Source: CAD feature listing. Evaluate the final solid. Frame: model axes, mm. Face numbers are marked on the shaded views. A direction names the side the tool comes from. Coordinates: 2 decimals unless noted, no trailing zeros. Loops run counter-clockwise (first coordinate to the right, second up) from the corner with the lowest first, then second, coordinate; pieces in that order, holes last. Notation, with made-up numbers: (40, 9) -> (54, 9) arc R17 ccw to (54, 28) -> close; hole circle Ø5 at (77, 71). An arc over 180 degrees is marked (long way). Answer as a JSON object with one key per item and string values. Group by question number.
from build123d import *

# Parameters (mm, degrees)
SKETCH_1_W          = 70.6
SKETCH_1_H          = 84.6
EXTRUDE_1_DEPTH     = 23
SKETCH_2_W          = 18
SKETCH_2_H          = 4.7
EXTRUDE_2_DEPTH     = 2
SKETCH_3_W          = 70.6
SKETCH_3_H          = 3.2
EXTRUDE_5_DEPTH     = 10
CUT_EXTRUDE_START   = -2
SKETCH_4_R          = 11
CUT_EXTRUDE_1_DEPTH = 115.979827321
EXTRUDE_START       = -2
EXTRUDE_1_2_DEPTH   = 2
DELETE_START        = 91
DELETE_FACE_1_DEPTH = 2
CUT_EXTRUDE_2_DEPTH = 43
EXTRUDE_START_2     = 24
EXTRUDE_6_DEPTH     = 2
FILLET_1_R          = 5


# Read off the part's stored shape, not the designer's step: 删除面1
with BuildPart() as part:
    # 草图1 → Extrude 1 (new body)
    with BuildSketch(Plane.XY):
        with Locations((-38.5, 47.5)):
            Rectangle(SKETCH_1_W, SKETCH_1_H)
    extrude(amount=-EXTRUDE_1_DEPTH)

    # 草图2 → 凸台-拉伸2 (add)
    with BuildSketch(Plane(origin=(0, 0, -23), x_dir=(-1, 0, 0), z_dir=(0, 0, -1))):
        with Locations((12.2, 2.85)):
            Rectangle(SKETCH_2_W, SKETCH_2_H)
        with Locations((64.8, 2.85)):
            Rectangle(SKETCH_2_W, SKETCH_2_H)
    extrude(amount=-EXTRUDE_2_DEPTH)

    # 草图3 → 凸台-拉伸5 (add)
    with BuildSketch(Plane(origin=(0, 0, -23), x_dir=(-1, 0, 0), z_dir=(0, 0, -1))):
        with Locations((38.5, 91.4)):
            Rectangle(SKETCH_3_W, SKETCH_3_H)
    extrude(amount=-EXTRUDE_5_DEPTH)

    # 草图4 → 切除-拉伸1 (cut, through all)
    with BuildSketch(Plane.XZ.offset(-5.2).offset(CUT_EXTRUDE_START)):
        with Locations((-60.8, -25)):
            Circle(SKETCH_4_R)
    extrude(amount=-CUT_EXTRUDE_1_DEPTH, mode=Mode.SUBTRACT)

    # 草图5 → Extrude 1 2 (add)
    with BuildSketch(Plane(origin=(0, 93, 0), x_dir=(1, 0, 0), z_dir=(0, 1, 0)).offset(EXTRUDE_START)):
        with BuildLine():
            ThreePointArc((-71.616653826, 23), (-60.8, 14), (-49.983346174, 23))
            Line((-49.983346174, 23), (-51.950010506, 23.363636364))
            ThreePointArc((-51.950010506, 23.363636364), (-60.8, 16), (-69.649989494, 23.363636364))
            Line((-69.649989494, 23.363636364), (-71.616653826, 23))
        make_face()
    extrude(amount=EXTRUDE_1_2_DEPTH)

    # Delete Face 1 outline → Delete Face 1 (cut)
    with BuildSketch(Plane(origin=(0, 0, 0), x_dir=(1, 0, 0), z_dir=(0, 1, 0)).offset(DELETE_START)):
        with BuildLine():
            ThreePointArc((-51.950010506, 23.363636364), (-51.985647631, 23.181431245), (-52.025035613, 23))
            Line((-52.025035613, 23), (-49.983346174, 23))
            Line((-49.983346174, 23), (-51.950010506, 23.363636364))
        make_face()
        with BuildLine():
            Line((-69.649989494, 23.363636364), (-71.616653826, 23))
            Line((-71.616653826, 23), (-69.574964387, 23))
            ThreePointArc((-69.574964387, 23), (-69.614352369, 23.181431245), (-69.649989494, 23.363636364))
        make_face()
    extrude(amount=DELETE_FACE_1_DEPTH, mode=Mode.SUBTRACT)

    # 草图6 → 切除-拉伸2 (cut)
    with BuildSketch(Plane(origin=(-3.2, 0, 0), x_dir=(0, 0, -1), z_dir=(1, 0, 0)).offset(CUT_EXTRUDE_START)):
        Polygon((23, 93), (15, 93), (15, 87.8), (2, 87.8), (2, 7.2), (23, 7.2), align=None)
    extrude(amount=-CUT_EXTRUDE_2_DEPTH, mode=Mode.SUBTRACT)

    # 草图7 → 凸台-拉伸6 (add)
    with BuildSketch(Plane.ZY.offset(5.2).offset(EXTRUDE_START_2)):
        Polygon((-23, 93), (-23, 7.2), (-2, 7.2), (-2, 87.8), (-15, 87.8), (-15, 93), align=None)
    extrude(amount=EXTRUDE_6_DEPTH)

    # 圆角1
    fillet_1_edges = [part.edges().sort_by_distance(p)[0] for p in [
        (-71.687482193, 93, -23),
        (-50.112517807, 93, -23),
        (-30.2, 93, -23),
        (-4.2, 93, -23),
    ]]
    fillet(fillet_1_edges, radius=FILLET_1_R)


solid = part.part
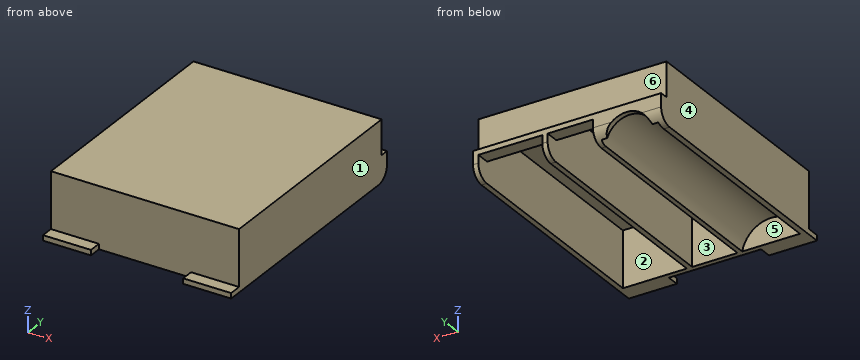
1. Mould query, pull axis Y, two halves, no side actions, for the marked faces 3, 4, 5 and 6. Classes: pulls with the +Y half, pulls with the -Y half, needs draft (parallel to the pull), parting line crosses it, or undercut.
2. Section query D-D on z = -17. Return loops of the section in (x, y).
3. Ray query, L1, parallel to X at y = 46, z = -5.25; L2, parallel to Y at x = -11.5, z = -9.5; L3, parallel to X at y = 66.5, z = -21. Return the intervals inside material, ascending.
4. Section query C-C on x = -42.5. Return loops of the section in (y, z).
5. Pin query (flat end, axial travel): pin 1 Ø2.5 at (x, y) = (-64.5, 3.5) entering from +Z; pin 2 Ø1.6 at (x, y) = (-36, 90.5) entering from -Z; pin 3 Ø1 at (x, y) = (-30.5, 90.5) entering from +Z. Return the tip coordinate at first contact, or that it passes through.
6. Section query A-A on z = -8. Return loops of the section in (x, y), then the cut area to 3 significant figures.
7. Reachability of the marked faces 1 and 2 from +Z, -Z, +X, -X, +Y, -Y: full face, straight path, thin tool, end or side. Return the list, or none.
8. Section query B-B on y = 67.5. Return loops of the section in (x, z).
Solved:
{
 "1": {"face 3": "undercut", "face 4": "needs draft", "face 5": "undercut", "face 6": "pulls with the +Y half"},
 "2": {"outline": "(-73.8, 5.2) -> (-3.2, 5.2) -> (-3.2, 93) -> (-5.2, 93) -> (-5.2, 7.2) -> (-29.2, 7.2) -> (-29.2, 93) -> (-31.2, 93) -> (-31.2, 7.2) -> (-48.2, 7.2) -> (-48.2, 93) -> (-56.68, 93) -> (-56.68, 91) -> (-53.25, 91) -> (-53.25, 7.2) -> (-68.35, 7.2) -> (-68.35, 91) -> (-64.92, 91) -> (-64.92, 93) -> (-73.8, 93) -> close"},
 "3": {"L1": "-73.8 to -48.2, -31.2 to -29.2, -5.2 to -3.2", "L2": "5.2 to 7.2, 87.8 to 89.8", "L3": "-73.8 to -71.05, -50.55 to -48.2, -31.2 to -29.2, -5.2 to -3.2"},
 "4": {"outline": "(5.2, -23) -> (7.2, -23) -> (7.2, -2) -> (87.8, -2) -> (87.8, -15) -> (93, -15) -> (93, -13) -> (89.8, -13) -> (89.8, 0) -> (5.2, 0) -> close"},
 "5": {"pin 1": "z = -21", "pin 2": "z = -15", "pin 3": "z = -13"},
 "6": {"outline": "(-73.8, 5.2) -> (-3.2, 5.2) -> (-3.2, 89.8) -> (-73.8, 89.8) -> close; hole (-48.2, 7.2) -> (-31.2, 7.2) -> (-31.2, 87.8) -> (-48.2, 87.8) -> close; hole (-29.2, 7.2) -> (-5.2, 7.2) -> (-5.2, 87.8) -> (-29.2, 87.8) -> close", "area": "2,670 mm^2"},
 "7": {"face 1": "+Z, -Z, +X, +Y, -Y", "face 2": "-Z"},
 "8": {"outline": "(-73.8, -23) -> (-71.62, -23) arc R11 cw to (-49.98, -23) -> (-48.2, -23) -> (-48.2, -2) -> (-31.2, -2) -> (-31.2, -23) -> (-29.2, -23) -> (-29.2, -2) -> (-5.2, -2) -> (-5.2, -23) -> (-3.2, -23) -> (-3.2, 0) -> (-73.8, 0) -> close"}
}
